```python
from build123d import *

# Parameters (mm, degrees)
F0_R          = 3.5
F1_DEPTH      = 56.35
F1_DEPTH_BACK = 1.5
F2_R          = 1
F3_DEPTH      = 2
F4_R          = 5
F5_R          = 5
F6_W          = 9.889290079
F6_H          = 18.65
F7_DEPTH      = 12.13642
F8_DEPTH      = 4
F9_R          = 1
F10_DEPTH     = 12.5
F11_R         = 1
F12_DEPTH     = 1.5
F13_R         = 1
F13_R_2       = 3.5
F14_DEPTH     = 1.71268
F15_R         = 4.5665029088
F16_DEPTH     = 1.5


with BuildPart() as f1:
    # F0 (on Top) → F1 (new body, two sides)
    with BuildSketch(Plane.XY) as f1_sk:
        Circle(F0_R)
    extrude(amount=F1_DEPTH)
    extrude(f1_sk.sketch, amount=-F1_DEPTH_BACK)

    # F2 (on Top) → F3 (join)
    with BuildSketch(Plane.XY):
        with BuildLine():
            Line((0, 4.5958375558), (-15.0020163562, 2.9683932874))
            ThreePointArc((-15.0020163562, 2.9683932874), (-16.902221013, 1.994188309), (-17.6658086413, 0))
            ThreePointArc((-17.6658086413, 0), (-16.902221013, -1.994188309), (-15.0020163562, -2.9683932874))
            Line((-15.0020163562, -2.9683932874), (0, -4.5958375558))
            Line((0, -4.5958375558), (15.0020163562, -2.9683932874))
            ThreePointArc((15.0020163562, -2.9683932874), (16.902221013, -1.994188309), (17.6658086413, 0))
            ThreePointArc((17.6658086413, 0), (16.902221013, 1.994188309), (15.0020163562, 2.9683932874))
            Line((15.0020163562, 2.9683932874), (0, 4.5958375558))
        make_face()
        with Locations((-14.68, 0)):
            Circle(F2_R, mode=Mode.SUBTRACT)
        with Locations((14.68, 0)):
            Circle(F2_R, mode=Mode.SUBTRACT)
    extrude(amount=-F3_DEPTH)

    # F4
    f4_edges = [f1.edges().sort_by_distance(p)[0] for p in [
        (0, 4.595838, -1),
    ]]
    fillet(f4_edges, radius=F4_R)

    # F5
    f5_edges = [f1.edges().sort_by_distance(p)[0] for p in [
        (0, -4.595838, -1),
    ]]
    fillet(f5_edges, radius=F5_R)

    # F6 (on Front) → F7 (cut)
    with BuildSketch(Plane.XZ):
        with Locations((-0.3122284543, 18.85)):
            Rectangle(F6_W, F6_H)
        with Locations((-0.3122284543, 37.5)):
            Rectangle(F6_W, F6_H)
    extrude(amount=-F7_DEPTH, mode=Mode.SUBTRACT)

    # F8 (add): a face of the model
    f8_faces = [f1.faces().sort_by_distance(p)[0] for p in [
        (0, 0, 56.35),
    ]]
    extrude(f8_faces, amount=F8_DEPTH)

    # F9 (on Front) → F10 (cut, symmetric)
    with BuildSketch(Plane.XZ):
        with Locations((0, 57.85)):
            Circle(F9_R)
    extrude(amount=F10_DEPTH, both=True, mode=Mode.SUBTRACT)

    # F11 (on face) → F12 (join)
    with BuildSketch(Plane(origin=(0, 0, -2), x_dir=(1, 0, 0), z_dir=(0, 0, -1))):
        with BuildLine():
            Line((-0.539244799, 4.5373393622), (-15.0020163562, 2.9683932874))
            ThreePointArc((-15.0020163562, 2.9683932874), (-17.6658086413, 0), (-15.0020163562, -2.9683932874))
            Line((-15.0020163562, -2.9683932874), (-0.539244799, -4.5373393622))
            ThreePointArc((-0.539244799, -4.5373393622), (0, -4.5665029088), (0.539244799, -4.5373393622))
            Line((0.539244799, -4.5373393622), (15.0020163562, -2.9683932874))
            ThreePointArc((15.0020163562, -2.9683932874), (17.6658086413, 0), (15.0020163562, 2.9683932874))
            Line((15.0020163562, 2.9683932874), (0.539244799, 4.5373393622))
            ThreePointArc((0.539244799, 4.5373393622), (0, 4.5665029088), (-0.539244799, 4.5373393622))
        make_face()
        with Locations((-14.68, 0)):
            Circle(F11_R, mode=Mode.SUBTRACT)
        with Locations((14.68, 0)):
            Circle(F11_R, mode=Mode.SUBTRACT)
    extrude(amount=F12_DEPTH)

    # F13 (on face) → F14 (cut)
    with BuildSketch(Plane.XY):
        with BuildLine():
            Line((0.539244799, -4.5373393622), (15.0020163562, -2.9683932874))
            ThreePointArc((15.0020163562, -2.9683932874), (17.6658086413, 0), (15.0020163562, 2.9683932874))
            Line((15.0020163562, 2.9683932874), (0.539244799, 4.5373393622))
            ThreePointArc((0.539244799, 4.5373393622), (0, 4.5665029088), (-0.539244799, 4.5373393622))
            Line((-0.539244799, 4.5373393622), (-15.0020163562, 2.9683932874))
            ThreePointArc((-15.0020163562, 2.9683932874), (-17.6658086413, 0), (-15.0020163562, -2.9683932874))
            Line((-15.0020163562, -2.9683932874), (-0.539244799, -4.5373393622))
            ThreePointArc((-0.539244799, -4.5373393622), (0, -4.5665029088), (0.539244799, -4.5373393622))
        make_face()
        with Locations((-14.68, 0)):
            Circle(F13_R, mode=Mode.SUBTRACT)
        Circle(F13_R_2, mode=Mode.SUBTRACT)
        with Locations((14.68, 0)):
            Circle(F13_R, mode=Mode.SUBTRACT)
    extrude(amount=-F14_DEPTH, mode=Mode.SUBTRACT)

    # F15 (on face) → F16 (join)
    with BuildSketch(Plane.XY.offset(-1.71268)):
        Circle(F15_R)
    extrude(amount=F16_DEPTH)


solid = f1.part
```
The listing builds one solid part. Answer for the finished solid, in the listing's coordinates (mm). A direction names the side the tool comes from. Give positions to 0.01 mm unless a question says otherwise; leave off trailing zeros. Order: outer loops, then holes, each group sorted by start corner. A loop starts at its lowest first (then second) coordinate and runs counter-clockwise, first axis right, second up.
1) Determine the mould class of faces 1 (the face through (-7.669, -3.764, -2.594)), 2 (the face through (-3.366, 3.086, -0.973)), 3 (the face through (-0.13, -0.05, 58.84)), 4 (the face through (7.669, 3.764, -2.594)) for opening direction X: pulls with the +X half, pulls with the -X half, needs draft (parallel to the pull), parting line crosses it, or undercut.
Reported:
face 1: pulls with the -X half
face 2: parting line crosses it
face 3: undercut
face 4: pulls with the +X half
2) Given P1, Ø2.5, axis at x = 0, z = 57.85, coming from the -Y side; P2, Ø2.5, axis at x = -14.68, y = 0, coming from the -Z side; P3, Ø4, axis at x = 14, y = -3.5, coming from the +Z side; P4, Ø4.5, axis at x = 6.5, y = 1, coming from the +Z side, each flat-ended and moving along its own axis, determine where each tip first touches the part or whether it passes through.
Reported:
P1: stops at y = -3.5
P2: stops at z = -3.5
P3: stops at z = -1.71
P4: stops at z = -0.21
3) Find section D-D on z = 50.5. Write down the section's boundary in (x, y), then the cut area to 3 significant figures.
Reported:
outline: circle Ø7 at (0, 0)
area: 38.5 mm2
4) For faces 5 (the face through (0, 0, -3.5)), 6 (the face through (-1.4, -3.4, -0.213)), 7 (the face through (0, 1, 9.525)), determine the directions among +Z, -Z, +X, -X, +Y, -Y from which every point of the face is accessible in a straight line to the end or side of a thin tool.
Reported:
face 5: -Z, +X, -X, +Y, -Y
face 6: +Z
face 7: +X, -X, +Y
5) Consider line 1 along X through (y, z) = (0, -2.85); line 2 along Z through (x, y) = (0, 0.25) (3 decimals); line 3 along Z through (x, y) = (0, -1). Determine where each line is inside the solid, lowest interval first.
Reported:
line 1: x = -17.67 to -15.68, -13.68 to 13.68, 15.68 to 17.67
line 2: z = -3.5 to 9.525, 46.825 to 56.85, 58.85 to 60.35
line 3: z = -3.5 to 56.85, 58.85 to 60.35
6) Find section C-C on z = 33. Write down the section's boundary in (x, y), then the cut area to 3 significant figures.
Reported:
outline: (-3.5, 0) arc R3.5 ccw to (3.5, 0) - close
area: 19.2 mm2
7) Find section B-B on x = -2. Write down the section's boundary in (y, z) (3 decimals), then the cut area to 3 significant figures.
Reported:
outline: (-4.379, -3.5) - (4.379, -3.5) - (4.379, -1.713) - (4.105, -1.713) - (4.105, -0.213) - (2.872, -0.213) - (2.872, 9.525) - (0, 9.525) - (0, 46.825) - (2.872, 46.825) - (2.872, 60.35) - (-2.872, 60.35) - (-2.872, -0.213) - (-4.105, -0.213) - (-4.105, -1.713) - (-4.379, -1.713) - close
area: 269 mm2
8) Find section A-A on y = 2. Write down the section's boundary in (x, z) (3 decimals).
Reported:
outline: (-16.897, -3.5) - (16.897, -3.5) - (16.897, -1.713) - (4.105, -1.713) - (4.105, -0.213) - (2.872, -0.213) - (2.872, 9.525) - (-2.872, 9.525) - (-2.872, -0.213) - (-4.105, -0.213) - (-4.105, -1.713) - (-16.897, -1.713) - close; (-2.872, 46.825) - (2.872, 46.825) - (2.872, 60.35) - (-2.872, 60.35) - close; hole circle Ø2 at (0, 57.85)
